The listing builds one solid part. Answer for the finished solid, in the listing's coordinates (mm). Coordinates: 2 decimals unless noted, no trailing zeros. Loops run counter-clockwise (first coordinate to the right, second up) from the corner with the lowest first, then second, coordinate; pieces in that order, holes last. Notation, with made-up numbers: M -6,-23 L 38,-23 A21 cw 38,-5 Z; hole C 48,55 d8. An arc over 180 degrees is marked long. Return JSON: item names as keys, results as strings. Group by question number.
1. Given P1, Ø3, axis at x = -6.275, z = -117, coming from the +Y side, flat-ended and moving along its own axis, determine where the tip first touches the part or whether it passes through.
2. Section A-A (z = -15) is taken. Write down the section's boundary in (x, y) (3 decimals), then the cut area to 3 significant figures.
3. Straight lines are drawn through the part: L1, parallel to Z at x = -6.5, y = 2.2; L2, parallel to Z at x = -8.5, y = 2.4. For each, find the intervals that lie inside material, in ascending order. Write a range as from..to.
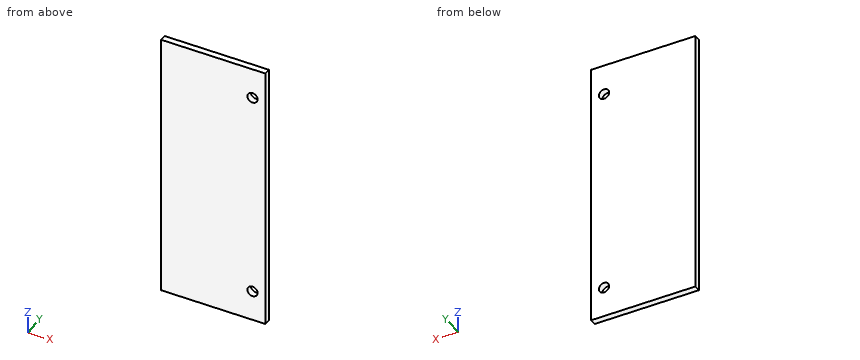
Autodesk Inventor part; units mm, degrees
ref_plane "YZ Plane" through (0, 0, 0) normal (1, 0, 0) x (0, 1, 0)
ref_plane "XZ Plane" through (0, 0, 0) normal (0, 1, 0) x (-1, 0, 0)
ref_plane "XY Plane" through (0, 0, 0) normal (0, 0, 1) x (1, 0, 0)
sketch "Sketch1" plane through (0, 0, 0) normal (0, 1, 0) x (-1, 0, 0)
  line L0 (0, 0) -> (50.75, 0)
  line L1 (50.75, 0) -> (50.75, -132)
  line L2 (50.75, -132) -> (0, -132)
  line L3 (0, -132) -> (0, 0)
  circle A0 centre (6.275, -15) radius 2.5
  circle A1 centre (6.275, -117) radius 2.5
  dimension "d0" = 50.75
  dimension "d1" = 132
  dimension "d4" = 5
  dimension "d5" = 5
  dimension "d6" = 6.275
  dimension "d7" = 6.275
  dimension "d8" = 15
  dimension "d9" = 15
extrude "Extrusion1" add sketch "Sketch1" along normal blind 3.1
properties part number "LoadCellPlate" material "Steel, Mild"
Worked out:
{
 "1": {"P1": "through"},
 "2": {"outline": "M -50.75,0 L -8.775,0 L -8.775,3.1 L -50.75,3.1 Z; M -3.775,0 L 0,0 L 0,3.1 L -3.775,3.1 Z", "area": "142 mm^2"},
 "3": {"L1": "-132..-119.49, -114.51..-17.49, -12.51..0", "L2": "-132..-118.14, -115.86..-16.14, -13.86..0"}
}
